from build123d import *

# Parameters (mm, degrees)
F1_DEPTH      = 114.6
F3_DEPTH      = 105.6
F5_DEPTH      = 8
F6_R          = 1.5
F7_DEPTH      = 20.401
F8_W          = 1
F8_H          = 1.8
F9_DEPTH      = 15.6
F10_T1_DEPTH  = 22.4
F10_T3_DEPTH  = 30.4
F10_T5_DEPTH  = 25.6
F10_T7_DEPTH  = 41.6
F10_T13_DEPTH = 30.6
F10_T17_DEPTH = 27.4
F10_T24_DEPTH = 30.6
F10_T28_DEPTH = 27.4


# Not quite as in the source:
# - a fillet or chamfer that OpenCascade refuses, or shapes differently, is made with other operations: its cross-section is extruded or revolved along the edge and cut away or added


with BuildPart() as f1:
    # F0 (on Front) → F1 (new body)
    with BuildSketch(Plane.XZ):
        Polygon((-15.8, 0), (0, 0), (15.8, 0), (15.8, 20.4), (11.8, 20.4), (11.8, 18.6), (12.8, 18.6), (12.8, 8), (11.8, 8), (11.8, 6.2), (12.8, 6.2), (12.8, 3), (3.4, 3), (3.4, 8), (2.75, 8), (0, 8), (-2.75, 8), (-3.4, 8), (-3.4, 3), (-12.8, 3), (-12.8, 6.2), (-11.8, 6.2), (-11.8, 8), (-12.8, 8), (-12.8, 18.6), (-11.8, 18.6), (-11.8, 20.4), (-15.8, 20.4), align=None)
        with BuildLine():
            ThreePointArc((0, 10.75), (-1.9445436483, 9.9445436483), (-2.75, 8))
            Line((-2.75, 8), (0, 8))
            Line((0, 8), (0, 10.75))
        make_face()
        with BuildLine():
            Line((0, 8), (2.75, 8))
            ThreePointArc((2.75, 8), (1.9445436483, 9.9445436483), (0, 10.75))
            Line((0, 10.75), (0, 8))
        make_face()
    extrude(amount=F1_DEPTH)

    # F2 (on face) → F3 (cut)
    with BuildSketch(Plane(origin=(0, 0, 0), x_dir=(-1, 0, 0), z_dir=(0, 1, 0))):
        with BuildLine():
            Line((-3.4, 8), (-3.4, 3))
            Line((-3.4, 3), (3.4, 3))
            Line((3.4, 3), (3.4, 8))
            Line((3.4, 8), (2.75, 8))
            ThreePointArc((2.75, 8), (0, 10.75), (-2.75, 8))
            Line((-2.75, 8), (-3.4, 8))
        make_face()
    extrude(amount=-F3_DEPTH, mode=Mode.SUBTRACT)

    # F4 (on face) → F5 (cut)
    with BuildSketch(Plane(origin=(0, -105.6, 0), x_dir=(-1, 0, 0), z_dir=(0, 1, 0))):
        with BuildLine():
            ThreePointArc((2.75, 8), (0, 10.75), (-2.75, 8))
            ThreePointArc((-2.75, 8), (-1.4940831044, 7.1353558864), (0, 6.8309673695))
            ThreePointArc((0, 6.8309673695), (1.4940831044, 7.1353558864), (2.75, 8))
        make_face()
    extrude(amount=-F5_DEPTH, mode=Mode.SUBTRACT)

    # F6 (on face) → F7 (cut, through all)
    with BuildSketch(Plane(origin=(0, 0, 0), x_dir=(1, 0, 0), z_dir=(0, 0, -1))):
        with Locations((0, 109.1)):
            Circle(F6_R)
    extrude(amount=-F7_DEPTH, mode=Mode.SUBTRACT)

    # F8 (on face) → F9 (cut)
    with BuildSketch(Plane(origin=(0, 0, 0), x_dir=(-1, 0, 0), z_dir=(0, 1, 0))):
        with Locations((-12.3, 19.5)):
            Rectangle(F8_W, F8_H)
        with Locations((-12.3, 7.1)):
            Rectangle(F8_W, F8_H)
        with Locations((12.3, 7.1)):
            Rectangle(F8_W, F8_H)
        with Locations((12.3, 19.5)):
            Rectangle(F8_W, F8_H)
    extrude(amount=-F9_DEPTH, mode=Mode.SUBTRACT)

    # F10: fillet of radius 2 on 6 edges, made by hand

    # F10_s2 → F10_t1 (cut)
    with BuildSketch(Plane.XY.offset(3)):
        with BuildLine():
            ThreePointArc((12.8, -2), (13.3857864376, -0.5857864376), (14.8, 0))
            Line((14.8, 0), (12.8, 0))
            Line((12.8, 0), (12.8, -2))
        make_face()
        with BuildLine():
            ThreePointArc((-12.8, -2), (-13.3857864376, -0.5857864376), (-14.8, 0))
            Line((-14.8, 0), (-12.8, 0))
            Line((-12.8, 0), (-12.8, -2))
        make_face()
    extrude(amount=F10_T1_DEPTH, mode=Mode.SUBTRACT)

    # F10_s4 → F10_t3 (cut)
    with BuildSketch(Plane.XY.offset(-5)):
        with BuildLine():
            ThreePointArc((15.8, -2), (15.2142135624, -0.5857864376), (13.8, 0))
            Line((13.8, 0), (15.8, 0))
            Line((15.8, 0), (15.8, -2))
        make_face()
        with BuildLine():
            ThreePointArc((-13.8, 0), (-15.2142135624, -0.5857864376), (-15.8, -2))
            Line((-15.8, -2), (-15.8, 0))
            Line((-15.8, 0), (-13.8, 0))
        make_face()
    extrude(amount=F10_T3_DEPTH, mode=Mode.SUBTRACT)

    # F10_s6 → F10_t5 (cut)
    with BuildSketch(Plane.YZ.offset(-12.8)):
        with BuildLine():
            ThreePointArc((-2, 3), (-0.5857864376, 2.4142135624), (0, 1))
            Line((0, 1), (0, 3))
            Line((0, 3), (-2, 3))
        make_face()
    extrude(amount=F10_T5_DEPTH, mode=Mode.SUBTRACT)

    # F10_s8 → F10_t7 (cut)
    with BuildSketch(Plane.YZ.offset(-20.8)):
        with BuildLine():
            ThreePointArc((-2, 0), (-0.5857864376, 0.5857864376), (0, 2))
            Line((0, 2), (0, 0))
            Line((0, 0), (-2, 0))
        make_face()
    extrude(amount=F10_T7_DEPTH, mode=Mode.SUBTRACT)


with BuildPart() as f10_tool11:
    # F10_s12 → F10_t13 (new body)
    with BuildSketch(Plane.YZ.offset(-12.8)):
        with BuildLine():
            ThreePointArc((-2, 3), (-0.5857864376, 2.4142135624), (0, 1))
            Line((0, 1), (0, 3))
            Line((0, 3), (-2, 3))
        make_face()
    extrude(amount=F10_T13_DEPTH)

    split(bisect_by=Plane.YZ.offset(12.8), keep=Keep.TOP)


with BuildPart() as f10_tool15:
    # F10_s16 → F10_t17 (new body)
    with BuildSketch(Plane.XY.offset(-2)):
        with BuildLine():
            ThreePointArc((12.8, -2), (13.3857864376, -0.5857864376), (14.8, 0))
            Line((14.8, 0), (12.8, 0))
            Line((12.8, 0), (12.8, -2))
        make_face()
    extrude(amount=F10_T17_DEPTH)

    split(bisect_by=Plane.XY.offset(3), keep=Keep.BOTTOM)


with BuildPart() as f10_tool11_1:
    add(f10_tool11.part)

    # F10_t19: intersect F10_tool15
    add(f10_tool15.part, mode=Mode.INTERSECT)


with BuildPart() as f1_1:
    add(f1.part)

    # F10_t9: cut F10_tool11
    add(f10_tool11_1.part, mode=Mode.SUBTRACT)


with BuildPart() as f10_tool22:
    # F10_s23 → F10_t24 (new body)
    with BuildSketch(Plane.YZ.offset(-17.8)):
        with BuildLine():
            ThreePointArc((-2, 3), (-0.5857864376, 2.4142135624), (0, 1))
            Line((0, 1), (0, 3))
            Line((0, 3), (-2, 3))
        make_face()
    extrude(amount=F10_T24_DEPTH)

    split(bisect_by=Plane.YZ.offset(-12.8), keep=Keep.BOTTOM)


with BuildPart() as f10_tool26:
    # F10_s27 → F10_t28 (new body)
    with BuildSketch(Plane.XY.offset(25.4)):
        with BuildLine():
            ThreePointArc((-12.8, -2), (-13.3857864376, -0.5857864376), (-14.8, 0))
            Line((-14.8, 0), (-12.8, 0))
            Line((-12.8, 0), (-12.8, -2))
        make_face()
    extrude(amount=-F10_T28_DEPTH)

    split(bisect_by=Plane.XY.offset(3), keep=Keep.BOTTOM)


with BuildPart() as f10_tool22_1:
    add(f10_tool22.part)

    # F10_t30: intersect F10_tool26
    add(f10_tool26.part, mode=Mode.INTERSECT)


with BuildPart() as f1_2:
    add(f1_1.part)

    # F10_t20: cut F10_tool22
    add(f10_tool22_1.part, mode=Mode.SUBTRACT)


solid = f1_2.part
Part model, mm, in its own coordinate system. A direction names the side the tool comes from. Coordinates: 2 decimals unless noted, no trailing zeros. Order: outer loops, then holes, each group sorted by start corner. A loop starts at its lowest first (then second) coordinate and runs counter-clockwise, first axis right, second up. Notation, with made-up numbers: (-9, 83.5) - (17, 83.5) arc R16 cw to (17, 94.5) - close; hole circle Ø11 at (9.25, 53). An arc over 180 degrees is marked (long way). Use CSV: the item, a comma, the result in double quotes.
Item 1: Drop flat-ended pins along their axis: P1, Ø1.1, axis at x = -12.5, y = -51, coming from the -Z side; P2, Ø6, axis at x = -0.5, y = -25.5, coming from the +Z side; P3, Ø0.5, axis at x = 12.5, z = 19.5, coming from the +Y side; P4, Ø1.1, axis at x = 12.5, z = 7, coming from the +Y side. Give the stop position or say it passes through.
Solved:
P1,"stops at z = 0"
P2,"stops at z = 3"
P3,"stops at y = -15.6"
P4,"stops at y = -1.03"
Item 2: Saw through at A-A on z = 4.5. Give the cut face in (x, y).
Solved:
outline,"(-15.8, -114.6) - (-12.8, -114.6) - (-12.8, -2) arc R2 ccw to (-14.3, -0.06) arc R2 ccw to (-15.8, -2) - close; (-3.4, -114.6) - (3.4, -114.6) - (3.4, -105.6) - (-3.4, -105.6) - close; (12.8, -114.6) - (15.8, -114.6) - (15.8, -2) arc R2 ccw to (14.3, -0.06) arc R2 ccw to (12.8, -2) - close; hole circle Ø3 at (0, -109.1)"
Item 3: Saw through at C-C on z = 14.25. Give the cut face in (x, y), and give its area (3 significant figures).
Solved:
outline,"(-15.8, -114.6) - (-12.8, -114.6) - (-12.8, -2) arc R2 ccw to (-14.3, -0.06) arc R2 ccw to (-15.8, -2) - close; (12.8, -114.6) - (15.8, -114.6) - (15.8, -2) arc R2 ccw to (14.3, -0.06) arc R2 ccw to (12.8, -2) - close"
area,"684 mm²"
Item 4: Probe probe 1 along X at (y, z) = (-109.1, 5.25); probe 2 along Z at (x, y) = (12.5, -55); probe 3 along X at (y, z) = (-22, 18). List the from-to ranges inside material, lowest first.
Solved:
probe 1,"x = -15.8 to -12.8, -3.4 to -1.5, 1.5 to 3.4, 12.8 to 15.8"
probe 2,"z = 0 to 3, 6.2 to 8, 18.6 to 20.4"
probe 3,"x = -15.8 to -12.8, 12.8 to 15.8"
Item 5: 3-axis set-ups, long thin cutter, end or side, ignore diameter. For faces 1 (the face through (3.4, -110, 5)), 2 (the face through (0.69, -107.77, 3.52)), 3 (the face through (-13.2, -0.8, 10.8)): which of +Z, -Z, +X, -X, +Y, -Y reach the whole face in a straight line?
Solved:
face 1,"+Z, +Y, -Y"
face 2,"+Z, -Z"
face 3,"+Z, +Y"
Item 6: Mould opens along X. For faces 4 (the face through (-15.8, -58, 10)), 5 (the face through (0, -58, 3)), 6 (the face through (-0.2, -0.8, 0.4)) say: +X half, -X half, draft (parallel to the pull), parting line (faces both ways), or undercut.
Solved:
face 4,"-X half"
face 5,"undercut"
face 6,"draft"
Item 7: Saw through at D-D on y = -76.5. Give the cut face in (x, z), and give its area (3 significant figures).
Solved:
outline,"(-15.8, 0) - (15.8, 0) - (15.8, 20.4) - (11.8, 20.4) - (11.8, 18.6) - (12.8, 18.6) - (12.8, 8) - (11.8, 8) - (11.8, 6.2) - (12.8, 6.2) - (12.8, 3) - (-12.8, 3) - (-12.8, 6.2) - (-11.8, 6.2) - (-11.8, 8) - (-12.8, 8) - (-12.8, 18.6) - (-11.8, 18.6) - (-11.8, 20.4) - (-15.8, 20.4) - close"
area,"206 mm²"
